Input: part model. Units: mm. Frame: model coordinates. Face numbers are marked on the shaded views. A direction names the side the tool comes from. Round coordinates to 2 decimals unless told otherwise and drop trailing zeros. Loops run counter-clockwise (first coordinate to the right, second up) from the corner with the lowest first, then second, coordinate; pieces in that order, holes last.
1) Ray query, line 1 along Y through (x, z) = (-119.25, 0); line 2 along Z through (x, y) = (-106.5, 61.5); line 3 along Y through (x, z) = (-117.5, 13.5). Return the intervals inside material, ascending.
2) Section A-A, the plane z = -9.5. Return loops of the section in (x, y), and give its area (3 significant figures).
3) Section C-C, the plane x = -86.5. Return loops of the section in (y, z), and give its area (3 significant figures).
4) Access query for the marked faces 4, 5 and 6. Directions: +Z, -Z, +X, -X, +Y, -Y. A direction counts if a zero-diameter tool reaches every point of the face in a straight line with its end or side. Return the directions, or none.
5) Section D-D, the plane z = 17.5. Return loops of the section in (x, y), and give its area (3 significant figures).
6) First-contact query: pin 1 (1.5 mm diameter, centred on y = 28.5, z = 0.5, fed in from +X); pin 2 (1.5 mm diameter, centred on x = -112, z = -10.5, fed in from +Y); pin 3 (7.5 mm diameter, centred on x = -127.5, z = 1, fed in from +Y). Flat tips, straight axial feed; report the tip coordinate or a pass-through.
7) Section B-B, the plane z = 0. Return loops of the section in (x, y).
8) Draft query along Z for the marked faces 1, 2 and 3. Return one class per face: pulls with the +Z half, pulls with the -Z half, needs draft (parallel to the pull), parting line crosses it, or undercut.
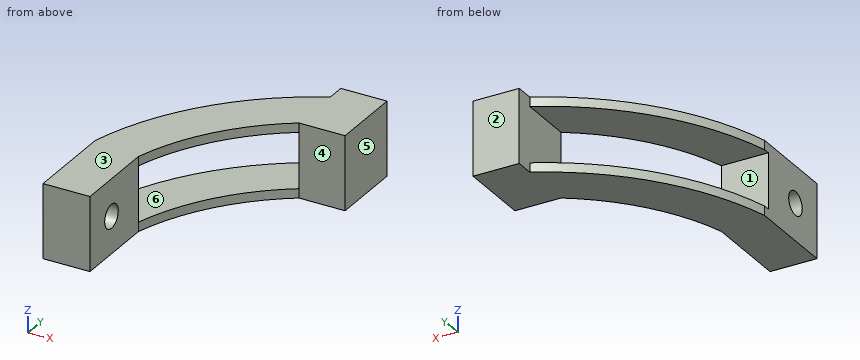
from build123d import *

# Parameters (mm, degrees)
SKETCH3_W                = 40
SKETCH3_H                = 45.541401669
BOSS_EXTRUDE2_DEPTH      = 300
BOSS_EXTRUDE2_DEPTH_BACK = 300
BOSS_EXTRUDE1_DEPTH      = 20
BOSS_EXTRUDE1_DEPTH_BACK = 20
CUT_EXTRUDE1_DEPTH       = 21
CUT_EXTRUDE1_DEPTH_BACK  = 21
SKETCH6_R                = 6.35
CUT_EXTRUDE3_DEPTH       = 464.230235913
SKETCH7_W                = 30
SKETCH7_H                = 500
CUT_EXTRUDE4_DEPTH       = 301
SKETCH9_W                = 717.699329224
SKETCH9_H                = 847.048890614
CUT_EXTRUDE6_DEPTH       = 21
CUT_EXTRUDE6_DEPTH_BACK  = 21
BOSS_EXTRUDE4_START      = -20
SKETCH11_W               = 25
SKETCH11_H               = 39.2080494
BOSS_EXTRUDE4_DEPTH      = 40
SKETCH15_W               = 300
SKETCH15_H               = 135
CUT_EXTRUDE9_DEPTH       = 21
CUT_EXTRUDE9_DEPTH_BACK  = 21


with BuildPart() as part:
    # Sketch3 → Boss-Extrude2 (new body, two sides)
    with BuildSketch(Plane(origin=(0, 0, 0), x_dir=(0, 0, -1), z_dir=(1, 0, 0))) as boss_extrude2_sk:
        with Locations((0, 10.070700834)):
            Rectangle(SKETCH3_W, SKETCH3_H)
    extrude(amount=BOSS_EXTRUDE2_DEPTH)
    extrude(boss_extrude2_sk.sketch, amount=-BOSS_EXTRUDE2_DEPTH_BACK)

    # Sketch2 → Boss-Extrude1 (add, two sides)
    with BuildSketch(Plane.XY) as boss_extrude1_sk:
        with BuildLine():
            Line((105.595237536, 0), (-143.695237536, 0))
            ThreePointArc((-143.695237536, 0), (0, 143.695237536), (143.695237536, 0))
            Line((143.695237536, 0), (105.595237536, 0))
        make_face()
    extrude(amount=BOSS_EXTRUDE1_DEPTH)
    extrude(boss_extrude1_sk.sketch, amount=-BOSS_EXTRUDE1_DEPTH_BACK)

    # Sketch4 → Cut-Extrude1 (cut, two sides)
    with BuildSketch(Plane.XY) as cut_extrude1_sk:
        with BuildLine():
            Line((113.645085948, 32.841401669), (113.645085948, -47.609700579))
            Line((113.645085948, -47.609700579), (-113.645085948, -47.609700579))
            Line((-113.645085948, -47.609700579), (-113.645085948, 32.841401669))
            ThreePointArc((-113.645085948, 32.841401669), (0, 118.295237536), (113.645085948, 32.841401669))
        make_face()
    extrude(amount=CUT_EXTRUDE1_DEPTH, mode=Mode.SUBTRACT)
    extrude(cut_extrude1_sk.sketch, amount=-CUT_EXTRUDE1_DEPTH_BACK, mode=Mode.SUBTRACT)

    # Sketch6 → Cut-Extrude3 (cut, through all)
    with BuildSketch(Plane.ZY.offset(163.230235913)):
        with Locations((0, 7.441401669)):
            Circle(SKETCH6_R)
    extrude(amount=-CUT_EXTRUDE3_DEPTH, mode=Mode.SUBTRACT)

    # Sketch7 → Cut-Extrude4 (cut, through all)
    with BuildSketch(Plane(origin=(0, 0, 0), x_dir=(0, 0, -1), z_dir=(1, 0, 0))):
        with Locations((0, 282.841401669)):
            Rectangle(SKETCH7_W, SKETCH7_H)
    extrude(amount=-CUT_EXTRUDE4_DEPTH, mode=Mode.SUBTRACT)

    # Sketch9 → Cut-Extrude6 (cut, two sides)
    with BuildSketch(Plane.XY) as cut_extrude6_sk:
        with Locations((318.769664612, 189.175554693)):
            Rectangle(SKETCH9_W, SKETCH9_H)
    extrude(amount=CUT_EXTRUDE6_DEPTH, mode=Mode.SUBTRACT)
    extrude(cut_extrude6_sk.sketch, amount=-CUT_EXTRUDE6_DEPTH_BACK, mode=Mode.SUBTRACT)

    # Sketch11 → Boss-Extrude4 (add)
    with BuildSketch(Plane.XY.offset(BOSS_EXTRUDE4_START)):
        with Locations((-52.58, 118.388420349)):
            Rectangle(SKETCH11_W, SKETCH11_H)
    extrude(amount=BOSS_EXTRUDE4_DEPTH)

    # Sketch15 → Cut-Extrude9 (cut, two sides)
    with BuildSketch(Plane.XY) as cut_extrude9_sk:
        with Locations((-289.045085948, 35.220701391)):
            Rectangle(SKETCH15_W, SKETCH15_H)
    extrude(amount=CUT_EXTRUDE9_DEPTH, mode=Mode.SUBTRACT)
    extrude(cut_extrude9_sk.sketch, amount=-CUT_EXTRUDE9_DEPTH_BACK, mode=Mode.SUBTRACT)


solid = part.part
Final values:
1. line 1: y = -12.7 to 1.09, 13.79 to 32.84
1. line 2: z = -20 to -15, 15 to 20
1. line 3: y = -12.7 to 32.84
2. outline: (-139.05, -12.7) - (-113.65, -12.7) - (-113.65, 32.84) - (-139.05, 32.84) - close; (-65.08, 98.78) - (-40.08, 98.78) - (-40.08, 137.99) - (-65.08, 137.99) - close
2. area: 2,140 mm2
3. outline: (80.69, -20) - (114.74, -20) - (114.74, -15) - (80.69, -15) - close; (80.69, 15) - (114.74, 15) - (114.74, 20) - (80.69, 20) - close
3. area: 340 mm2
4. face 4: +Z, -Z, +X, -Y
4. face 5: +Z, -Z, +X, +Y, -Y
4. face 6: -X, +Y
5. outline: (-139.05, -12.7) - (-113.65, -12.7) - (-113.65, 32.84) arc R118.3 cw to (-65.08, 98.78) - (-40.08, 98.78) - (-40.08, 137.99) - (-65.08, 137.99) - (-65.08, 128.11) arc R143.7 ccw to (-139.05, 36.26) - close
5. area: 4,790 mm2
6. pin 1: stops at x = -113.65
6. pin 2: passes through
6. pin 3: stops at y = 32.84
7. outline: (-139.05, -12.7) - (-113.65, -12.7) - (-113.65, 1.09) - (-139.05, 1.09) - close; (-139.05, 13.79) - (-113.65, 13.79) - (-113.65, 32.84) - (-139.05, 32.84) - close; (-65.08, 98.78) - (-40.08, 98.78) - (-40.08, 137.99) - (-65.08, 137.99) - close
8. face 1: undercut
8. face 2: needs draft
8. face 3: pulls with the +Z half
